Study the drawing (mm; zero at the part's minimum x, y, z) and answer. Round coordinates to 2 decimals unless told otherwise and drop trailing zeros. Order: outer loops, then holes, each group sorted by start corner. A loop starts at its lowest first (then second) coordinate and runs counter-clockwise, first axis right, second up. Notation, with made-up numbers: M 82.25,46.25 L 111.25,46.25 A20 ccw 111.25,61.25 Z; hole C 65,89.5 d7. An arc over 180 degrees is marked long. Put each result on its own line as item: value. Start each with the question number.
1. Consider line 1 (Y direction, x = 2.5, z = 27); line 2 (Z direction, x = 2.75, y = 6); line 3 (Y direction, x = 1.5, z = 5). Determine where each line is inside the solid, lowest interval first.
2. The part is cut by section B-B (z = 30). Count the separate pieces of the cut face and the enclosed holes in it, then the cut area to 3 significant figures.
3. Each of these flat-tipped pins is pushed along its axis until it touches: pin 1 Ø3 at (x, z) = (2, 52) entering from +Y; pin 2 Ø3 at (y, z) = (45.24, 30.16) entering from +X; pin 3 Ø1.9 at (x, y) = (2.5, 31.5) entering from +Z; pin 4 Ø1 at (x, y) = (2, 30) entering from -Z. Where does it stop, or does it pass through?
4. The part is cut by section D-D (y = 54.5). Give the vertices of the cut face in (x, z).
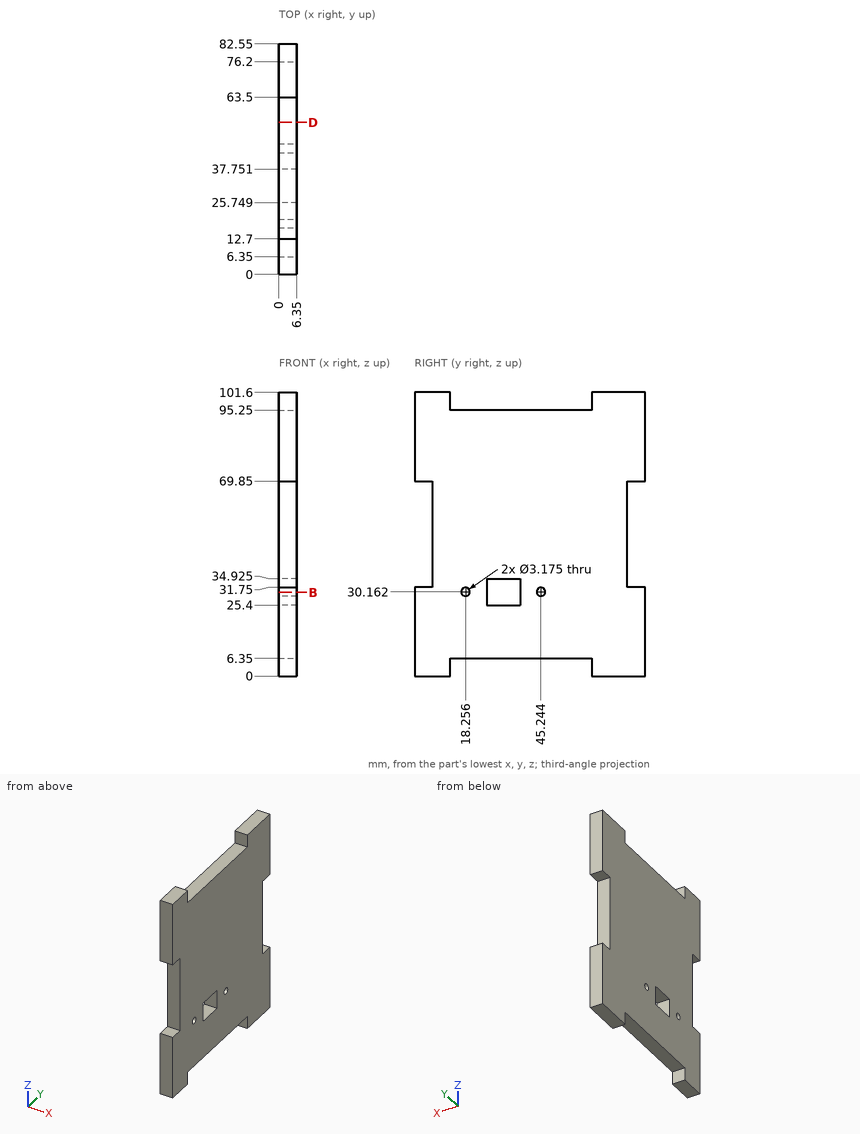
Resolved:
1. line 1: 0 to 25.75, 37.75 to 82.55
1. line 2: 0 to 31.75, 69.85 to 101.6
1. line 3: 0 to 12.7, 63.5 to 82.55
2. separate pieces: 4
2. enclosed holes: 0
2. area: 408 mm2
3. pin 1: y = 76.2
3. pin 2: through
3. pin 3: z = 95.25
3. pin 4: z = 6.35
4. outline: M 0,6.35 L 6.35,6.35 L 6.35,95.25 L 0,95.25 Z
